from build123d import *

# Parameters (mm, degrees)
F1_DEPTH = 25.4


with BuildPart() as f1:
    # F0 (on Front) → F1 (new body)
    with BuildSketch(Plane.XZ):
        with BuildLine():
            ThreePointArc((-77.954433, 36.849992), (-83.324328, 37.92253), (-88.679372, 39.066919))
            ThreePointArc((-88.679372, 39.066919), (-129.049346, 1.034601), (-88.679372, -36.997717))
            ThreePointArc((-88.679372, -36.997717), (-87.773383, -36.921511), (-86.867329, -36.846095))
            ThreePointArc((-86.867329, -36.846095), (-63.305117, -25.183839), (-52.905742, -1.037637))
            Line((-52.905742, -1.037637), (-59.431807, -2.8004))
            ThreePointArc((-59.431807, -2.8004), (-122.691774, 0.341231), (-59.62933, 6.242203))
            Line((-59.62933, 6.242203), (-53.462953, 7.844913))
            ThreePointArc((-53.462953, 7.844913), (-61.838966, 25.614996), (-77.954433, 36.849992))
        make_face()
        with BuildLine():
            ThreePointArc((-77.954433, 36.849992), (-83.236831, 38.345821), (-88.679372, 39.066919))
            ThreePointArc((-88.679372, 39.066919), (-83.324328, 37.92253), (-77.954433, 36.849992))
        make_face()
        with BuildLine():
            ThreePointArc((-86.867329, -36.846095), (-87.773383, -36.921511), (-88.679372, -36.997717))
            ThreePointArc((-88.679372, -36.997717), (-87.772445, -36.932718), (-86.867329, -36.846095))
        make_face()
        with BuildLine():
            ThreePointArc((-46.762083, 32.077556), (-62.404336, 34.162613), (-77.954433, 36.849992))
            ThreePointArc((-77.954433, 36.849992), (-61.838966, 25.614996), (-53.462953, 7.844913))
            Line((-53.462953, 7.844913), (-46.762083, 9.586544))
            Line((-46.762083, 9.586544), (-46.762083, 32.077556))
        make_face()
        with BuildLine():
            ThreePointArc((-52.905742, -1.037637), (-63.305117, -25.183839), (-86.867329, -36.846095))
            ThreePointArc((-86.867329, -36.846095), (-3.539116, -33.292767), (79.806603, -36.408574))
            ThreePointArc((79.806603, -36.408574), (57.814967, -23.63398), (48.761331, 0.132676))
            Line((48.761331, 0.132676), (20.909883, 6.46305))
            Line((20.909883, 6.46305), (-25.136846, 6.46305))
            Line((-25.136846, 6.46305), (-52.905742, -1.037637))
        make_face()
        with BuildLine():
            ThreePointArc((87.74957, -37.054793), (83.778703, -36.724097), (79.806603, -36.408574))
            ThreePointArc((79.806603, -36.408574), (83.761144, -36.939929), (87.74957, -37.054793))
        make_face()
        with BuildLine():
            ThreePointArc((48.761331, 0.132676), (57.814967, -23.63398), (79.806603, -36.408574))
            ThreePointArc((79.806603, -36.408574), (83.778703, -36.724097), (87.74957, -37.054793))
            ThreePointArc((87.74957, -37.054793), (124.950654, 1.034601), (87.74957, 39.123995))
            ThreePointArc((87.74957, 39.123995), (79.575458, 37.401709), (71.367851, 35.846852))
            ThreePointArc((71.367851, 35.846852), (57.209182, 24.971876), (49.558952, 8.840943))
            Line((49.558952, 8.840943), (55.758314, 7.463354))
            ThreePointArc((55.758314, 7.463354), (118.534221, -1.018226), (55.188695, -1.328204))
            Line((55.188695, -1.328204), (48.761331, 0.132676))
        make_face()
        with BuildLine():
            ThreePointArc((71.367851, 35.846852), (79.575458, 37.401709), (87.74957, 39.123995))
            ThreePointArc((87.74957, 39.123995), (79.376876, 38.394374), (71.367851, 35.846852))
        make_face()
        with BuildLine():
            ThreePointArc((49.558952, 8.840943), (57.209182, 24.971876), (71.367851, 35.846852))
            ThreePointArc((71.367851, 35.846852), (56.790326, 33.510204), (42.137917, 31.701597))
            Line((42.137917, 31.701597), (42.137917, 10.490005))
            Line((42.137917, 10.490005), (49.558952, 8.840943))
        make_face()
    extrude(amount=F1_DEPTH)


solid = f1.part
Model file for the job. Use its own axes, mm. A direction names the side the tool comes from. Give positions to 0.01 mm unless a question says otherwise; leave off trailing zeros. Write each loop counter-clockwise with the first axis right and the second up, starting at its lowest first coordinate (ties: lowest second). Pieces come first, ordered by that corner, then holes. Notation, with made-up numbers: (57.5, 59.25) - (92.5, 59.25) arc R31 cw to (92.5, 87.25) - close; hole circle Ø5 at (11.5, -13). An arc over 180 degrees is marked (long way). Answer as CSV lines item,"result".
1. Band-saw the part on B-B (x = -105). Write the cut outline in (y, z), and give its area (3 significant figures).
Responses:
outline,"(-25.4, -34.38) - (0, -34.38) - (0, -27.44) - (-25.4, -27.44) - close; (-25.4, 29.51) - (0, 29.51) - (0, 36.45) - (-25.4, 36.45) - close"
area,"353 mm2"
2. Band-saw the part on C-C (z = -12.5). Write the cut outline in (x, y).
Responses:
outline,"(-126.56, -25.4) - (-119.67, -25.4) - (-119.67, 0) - (-126.56, 0) - close; (-62.23, -25.4) - (58.13, -25.4) - (58.13, 0) - (-62.23, 0) - close; (115.57, -25.4) - (122.47, -25.4) - (122.47, 0) - (115.57, 0) - close"
3. Two-plate mould, pull along Z, no slides. Class faces 3 (the face through (56.99, -12.52, 33.54)), 4 (the face through (-122.635, -12.522, -0.99)), 5 (the face through (-129.04, -12.52, 1.9)): +Z half, -Z half, draft (parallel to the pull), parting line (faces both ways), or undercut.
Responses:
face 3,"+Z half"
face 4,"undercut"
face 5,"parting line"
4. 3-axis set-ups, long thin cutter, end or side, ignore diameter. For faces 1 (the face through (-62.19, -12.52, 34.13)), 2 (the face through (-4, 0, -7)): which of +Z, -Z, +X, -X, +Y, -Y reach the whole face in a straight line?
Responses:
face 1,"+Z, +Y, -Y"
face 2,"+Z, -Z, +X, -X, +Y"
5. Band-saw the part on A-A (z = 17.5). Write the cut outline in (x, y), and give its area (3 significant figures).
Responses:
outline,"(-125.31, -25.4) - (-118.1, -25.4) - (-118.1, 0) - (-125.31, 0) - close; (-63.8, -25.4) - (-46.76, -25.4) - (-46.76, 0) - (-63.8, 0) - close; (42.14, -25.4) - (59.7, -25.4) - (59.7, 0) - (42.14, 0) - close; (114, -25.4) - (121.21, -25.4) - (121.21, 0) - (114, 0) - close"
area,"1,250 mm2"
6. Drill centre lines: L1, parallel to Z at x = -90.5, y = -23; L2, parallel to X at y = -22.5, z = -17.5; L3, parallel to X at y = -22.25, z = 28. Where is each one in solid material? Low to high. Write a range as [from, to].
Responses:
L1,"z = [-37.06, -30.71], [32.78, 39.13]"
L2,"x = [-124.24, -116.73], [-65.17, 61.07], [112.63, 120.14]"
L3,"x = [-117.87, -107.71], [-74.19, -46.76], [42.14, 70.09], [103.61, 113.77]"
7. Pin check, flat tips, straight feed: pin 1 (6 mm diameter, centred on y = -9.5, z = -22.5, fed in from -X); pin 2 (6 mm diameter, centred on x = -76.5, y = -7.5, fed in from +Z); pin 3 (10 mm diameter, centred on x = -80.5, y = -18.5, fed in from +Z). Stop position of each tip, or through.
Responses:
pin 1,"stops at x = -123.04"
pin 2,"stops at z = 37.37"
pin 3,"stops at z = 38.74"
8. Band-saw the part on D-D (y = -4). Write the cut outline in (x, z), and give its area (3 significant figures).
Responses:
outline,"(-88.68, -37) arc R38.1 ccw to (-86.87, -36.85) arc R1043.04 cw to (79.81, -36.41) arc R38.1 ccw to (87.75, -37.05) arc R38.1 ccw (long way) to (71.37, 35.85) arc R408.69 cw to (42.14, 31.7) - (42.14, 10.49) - (55.76, 7.46) arc R31.75 cw (long way) to (55.19, -1.33) - (20.91, 6.46) - (-25.14, 6.46) - (-59.43, -2.8) arc R31.75 cw (long way) to (-59.63, 6.24) - (-46.76, 9.59) - (-46.76, 32.08) arc R408.69 cw to (-77.95, 36.85) arc R38.1 ccw to (-88.68, 39.07) arc R38.1 ccw (long way) to start"
area,"7,740 mm2"
